Design review of the part built by this model. Coordinates are the model's own, in mm. A direction names the side the tool comes from. Round coordinates to 2 decimals unless told otherwise and drop trailing zeros. Loops run counter-clockwise (first coordinate to the right, second up) from the corner with the lowest first, then second, coordinate; pieces in that order, holes last. Notation, with made-up numbers: (49, 5.5) - (65, 5.5) arc R11 ccw to (65, 21.5) - close; hole circle Ø7 at (20.5, -20). An arc over 180 degrees is marked (long way). Use one line per item in the form item = value. Start each with the question number.
(1) Machinability: for faces 1 (the flat face through (-12.5, 49, 12)), 2 (the flat face through (-5.4, 8.2, 6)), 3 (the cylindrical face through (-27.591, 151.026, 19.944)), 4 (the flat face through (-35.5, 115, 12)), 5 (the flat face through (-20, 160, 8)), which of the approach directions +Z, -Z, +X, -X, +Y, -Y give a long, thin tool a straight path to every point of the face, cutting with its end or side? Answer none if there is none.
(2) For pin 1 (4 mm diameter, centred on x = -21, z = 17.5, fed in from -Y); pin 2 (12 mm diameter, centred on y = 44, z = 7, fed in from -X); pin 3 (2.5 mm diameter, centred on x = 1, z = 12.5, fed in from +Y); pin 4 (20 mm diameter, centred on x = -1.5, y = -0.5, fed in from +Z), all flat-tipped, find the tip position at first contact; note any pin that passes through.
(3) We need section C-C, the plane x = -7.5. Write out the cut boundary in (y, z).
(4) The part is to be moulded in two halves that separate along X. For faces 6 (the cylindrical face through (0.6, 155.7, 6.5)), 7 (the flat face through (-5, 88, 24)), 8 (the cylindrical face through (4.38, -8.43, 2.96)), say which applies: released by +X, released by -X, zero draft, split by the parting line, or undercut.
(5) Wall thickness on probe 1 along Y at (x, z) = (-25, 16.25); probe 2 along Y at (x, z) = (-22.5, 16.75); probe 3 along X at (y, z) = (114.5, 9): over which ranges is each line inside the solid? List them lowest first. Write a range as [from, to].
(6) We need section B-B, the plane y = 4.5. Write out the cut boundary in (x, z).
(7) We need section A-A, the plane x = 0. Write out the cut boundary in (y, z).
from build123d import *

# Parameters (mm, degrees)
CROQUIS2_R                 = 12.5
CROQUIS2_R_2               = 9.5
SALIENTE_EXTRUIR1_DEPTH    = 24
CORTAR_EXTRUIR3_DEPTH      = 191.437747955
CORTAR_EXTRUIR3_DEPTH_BACK = 191.437747955
CROQUIS5_W                 = 8
CROQUIS5_H                 = 49.434743854
CORTAR_EXTRUIR4_DEPTH      = 191.437747955
CORTAR_EXTRUIR4_DEPTH_BACK = 191.437747955
CROQUIS6_W                 = 12
CROQUIS6_H                 = 25
CORTAR_EXTRUIR5_DEPTH      = 159.265939688
CORTAR_EXTRUIR5_DEPTH_BACK = 159.265939688
CROQUIS7_W                 = 14.533349016
CROQUIS7_H                 = 8


with BuildPart() as part:
    # Croquis2 → Saliente-Extruir1 (new body)
    # profile 1 of 4: a face of its own
    with BuildSketch(Plane.XY):
        with Locations((-37.533349016, 172.653405471)):
            Circle(CROQUIS2_R)
        with Locations((-37.533349016, 172.653405471)):
            Circle(CROQUIS2_R_2, mode=Mode.SUBTRACT)
    # profile 2 of 4: a face of its own
    with BuildSketch(Plane.XY):
        with BuildLine():
            Line((-12.5, 58.855421297), (-12.5, 0))
            ThreePointArc((-12.5, 0), (0, 12.5), (12.5, 0))
            Line((12.5, 0), (12.5, 115))
            ThreePointArc((12.5, 115), (0.265693313, 156.217157525), (-32.475079629, 184.08423706))
            ThreePointArc((-32.475079629, 184.08423706), (-27.057701844, 179.473289366), (-25.033349016, 172.653405471))
            ThreePointArc((-25.033349016, 172.653405471), (-30.713465121, 162.1777583), (-42.591618403, 161.222573883))
            ThreePointArc((-42.591618403, 161.222573883), (-27.406897086, 150.843693068), (-16.941222141, 135.718661617))
            ThreePointArc((-16.941222141, 135.718661617), (-17.037727548, 131.417260647), (-20.439743892, 128.783319041))
            Line((-20.439743892, 128.783319041), (-27.655370554, 127.214704549))
            ThreePointArc((-27.655370554, 127.214704549), (-17.155961879, 124.732474812), (-12.5, 115))
            ThreePointArc((-12.5, 115), (-16.161165235, 106.161165235), (-25, 102.5))
            Line((-25, 102.5), (-17.5, 102.5))
            ThreePointArc((-17.5, 102.5), (-13.964466094, 101.035533906), (-12.5, 97.5))
            Line((-12.5, 97.5), (-12.5, 58.855421297))
        make_face()
    # profile 3 of 4: a face of its own
    with BuildSketch(Plane.XY):
        with Locations((-25, 115)):
            Circle(CROQUIS2_R)
        with Locations((-25, 115)):
            Circle(CROQUIS2_R_2, mode=Mode.SUBTRACT)
    # profile 4 of 4: a face of its own
    with BuildSketch(Plane.XY):
        Circle(CROQUIS2_R)
        Circle(CROQUIS2_R_2, mode=Mode.SUBTRACT)
    extrude(amount=SALIENTE_EXTRUIR1_DEPTH)

    # Croquis5 → Cortar-Extruir3 (cut, two sides: drawn at the far end of the back side and taken through both)
    with BuildSketch(Plane.ZY.offset(12.5).offset(-CORTAR_EXTRUIR3_DEPTH_BACK)):
        with Locations((12, 160.436033544)):
            Rectangle(CROQUIS5_W, CROQUIS5_H)
    extrude(amount=CORTAR_EXTRUIR3_DEPTH + CORTAR_EXTRUIR3_DEPTH_BACK, mode=Mode.SUBTRACT)

    # Croquis6 → Cortar-Extruir4 (cut, two sides: drawn at the far end of the back side and taken through both)
    with BuildSketch(Plane.ZY.offset(12.5).offset(-CORTAR_EXTRUIR4_DEPTH_BACK)):
        with Locations((12, 0)):
            Rectangle(CROQUIS6_W, CROQUIS6_H)
    extrude(amount=CORTAR_EXTRUIR4_DEPTH + CORTAR_EXTRUIR4_DEPTH_BACK, mode=Mode.SUBTRACT)

    # Croquis7 → Cortar-Extruir5 (cut, two sides: drawn at the far end of the back side and taken through both)
    with BuildSketch(Plane(origin=(0, 135.718661617, 0), x_dir=(1, 0, 0), z_dir=(0, 1, 0)).offset(-CORTAR_EXTRUIR5_DEPTH_BACK)):
        with Locations((-42.766674508, -12)):
            Rectangle(CROQUIS7_W, CROQUIS7_H)
    extrude(amount=CORTAR_EXTRUIR5_DEPTH + CORTAR_EXTRUIR5_DEPTH_BACK, mode=Mode.SUBTRACT)


solid = part.part
Data:
q1.face_1 = +Z, -Z, -X, -Y
q1.face_2 = +X, -X, -Y
q1.face_3 = +Z, -Z, -X
q1.face_4 = -X, +Y, -Y
q1.face_5 = +X, -X, +Y
q2.pin_1 = 102.5
q2.pin_2 = -12.5
q2.pin_3 = 135.72
q2.pin_4 = 24
q3.outline = (-10, 0) - (-5.83, 0) - (-5.83, 6) - (-10, 6) - close; (-10, 18) - (-5.83, 18) - (-5.83, 24) - (-10, 24) - close; (5.83, 0) - (166.2, 0) - (166.2, 8) - (135.72, 8) - (135.72, 16) - (166.2, 16) - (166.2, 24) - (5.83, 24) - (5.83, 18) - (12.5, 18) - (12.5, 6) - (5.83, 6) - close
q4.face_6 = released by +X
q4.face_7 = zero draft
q4.face_8 = undercut
q5.probe_1 = [102.5, 105.5], [124.5, 127.79], [148.28, 180.27]
q5.probe_2 = [102.5, 105.83], [124.17, 128.34], [145.18, 178.74]
q5.probe_3 = [-35.5, -34.49], [-15.51, 12.5]
q6.outline = (-12.5, 0) - (-8.37, 0) - (-8.37, 6) - (-12.5, 6) - close; (-12.5, 18) - (-8.37, 18) - (-8.37, 24) - (-12.5, 24) - close; (8.37, 0) - (12.5, 0) - (12.5, 6) - (8.37, 6) - close; (8.37, 18) - (12.5, 18) - (12.5, 24) - (8.37, 24) - close
q7.outline = (-12.5, 0) - (-9.5, 0) - (-9.5, 6) - (-12.5, 6) - close; (-12.5, 18) - (-9.5, 18) - (-9.5, 24) - (-12.5, 24) - close; (9.5, 0) - (156.62, 0) - (156.62, 8) - (135.72, 8) - (135.72, 16) - (156.62, 16) - (156.62, 24) - (9.5, 24) - (9.5, 18) - (12.5, 18) - (12.5, 6) - (9.5, 6) - close
